Here's how the part is built. I have some questions about the finished solid (model axes, mm). A direction names the side the tool comes from. Coordinates: 2 decimals unless noted, no trailing zeros. Write each loop counter-clockwise with the first axis right and the second up, starting at its lowest first coordinate (ties: lowest second). Pieces come first, ordered by that corner, then holes.
Item 1: For faces 1 (the face through (0.37, 66.05, 0.01)), 2 (the face through (-6.3, 4.7, 12.5)), 3 (the face through (40, 41.5, 0)), which set-ups out of +Z, -Z, +X, -X, +Y, -Y let a thin tool reach every point of the face, with its end or its side?
Item 2: If we section it at B-B (x = -24): Please give me the cut outline in (y, z), then the cut area to 3 significant figures.
Item 3: If I drill on line 1 (Y direction, x = 2.5, z = -5); line 2 (X direction, y = 7, z = -7); line 3 (Y direction, x = -12, z = -1.75), over which ranges is the centre line in solid material (lowest first)?
Item 4: If we section it at D-D (y = 12.5): Please give me the cut outline in (x, z).
Item 5: I'm going to push flat-ended pins straight in: pin 1 Ø8 at (x, z) = (0, 2.5) entering from +Y; pin 2 Ø5 at (y, z) = (59, 0) entering from -X; pin 3 Ø10 at (x, y) = (13, 58.5) entering from +Z. Where does each tip first touch, or does it pass through?
Item 6: We'd pull the mould along Y, two halves only. Please class faces 4 (the face through (41.25, 4, 0)), 5 (the face through (1, 5, 0)), 6 (the face through (-1, 0, 0)): +Y half, -Y half, draft (parallel to the pull), parting line (faces both ways), or undercut.
Item 7: If we section it at C-C (z = -8): Please give me the cut outline in (x, y).
Item 8: If we section it at A-A (x = 0): Please give me the cut outline in (y, z), then the cut area to 3 significant figures.
from build123d import *

# Parameters (mm, degrees)
SKETCH1_W               = 82.5
SKETCH1_H               = 25
BOSS_EXTRUDE1_DEPTH     = 5
SKETCH2_W               = 5
SKETCH2_H               = 25
BOSS_EXTRUDE2_DEPTH     = 39
SKETCH3_W               = 82.5
SKETCH3_H               = 25
BOSS_EXTRUDE3_DEPTH     = 5
BOSS_EXTRUDE4_DEPTH     = 2.5
SKETCH5_W               = 2.5
SKETCH5_H               = 39
BOSS_EXTRUDE5_DEPTH     = 25
CUT_EXTRUDE1_DEPTH      = 86.323912034
CUT_EXTRUDE1_DEPTH_BACK = 25
SKETCH6_W               = 5
SKETCH6_H               = 34
FILLET1_R               = 2
FILLET2_R               = 2


with BuildPart() as part:
    # Sketch1 → Boss-Extrude1 (new body)
    with BuildSketch(Plane(origin=(0, 0, 0), x_dir=(1, 0, 0), z_dir=(0, 1, 0))):
        Rectangle(SKETCH1_W, SKETCH1_H)
    extrude(amount=BOSS_EXTRUDE1_DEPTH)

    # Sketch2 → Boss-Extrude2 (add)
    with BuildSketch(Plane(origin=(0, 5, 0), x_dir=(1, 0, 0), z_dir=(0, 1, 0))):
        with Locations((-38.75, 0)):
            Rectangle(SKETCH2_W, SKETCH2_H)
    extrude(amount=BOSS_EXTRUDE2_DEPTH)

    # Sketch3 → Boss-Extrude3 (add)
    with BuildSketch(Plane(origin=(0, 44, 0), x_dir=(1, 0, 0), z_dir=(0, 1, 0))):
        Rectangle(SKETCH3_W, SKETCH3_H)
    extrude(amount=BOSS_EXTRUDE3_DEPTH)

    # Sketch4 → Boss-Extrude4 (add, symmetric)
    with BuildSketch(Plane.XY):
        with BuildLine():
            Line((-17.053024247, 49), (-21.381868864, 49))
            ThreePointArc((-21.381868864, 49), (0, 70.381868864), (21.381868864, 49))
            Line((21.381868864, 49), (17.053024247, 49))
            ThreePointArc((17.053024247, 49), (0, 66.053024247), (-17.053024247, 49))
        make_face()
    extrude(amount=BOSS_EXTRUDE4_DEPTH, both=True)

    # Sketch5 → Boss-Extrude5 (add)
    with BuildSketch(Plane.XY.offset(12.5)):
        with Locations((40, 24.5)):
            Rectangle(SKETCH5_W, SKETCH5_H)
    extrude(amount=-BOSS_EXTRUDE5_DEPTH)

    # Sketch6 → Cut-Extrude1 (cut, two sides: drawn at the far end of the back side and taken through both)
    with BuildSketch(Plane.XY.offset(12.5).offset(-CUT_EXTRUDE1_DEPTH_BACK)):
        with Locations((38.75, 24.5)):
            Rectangle(SKETCH6_W, SKETCH6_H)
    extrude(amount=CUT_EXTRUDE1_DEPTH + CUT_EXTRUDE1_DEPTH_BACK, mode=Mode.SUBTRACT)

    # Fillet1
    fillet1_edges = [part.edges().sort_by_distance(p)[0] for p in [
        (0, 70.381868864, -2.5),
        (0, 70.381868864, 2.5),
    ]]
    fillet(fillet1_edges, radius=FILLET1_R)

    # Fillet2
    fillet2_edges = [part.edges().sort_by_distance(p)[0] for p in [
        (0, 66.053024247, -2.5),
        (0, 66.053024247, 2.5),
    ]]
    fillet(fillet2_edges, radius=FILLET2_R)


solid = part.part
Answer list:
1. face 1: +Z, -Z
1. face 2: +Z, +X, -X, +Y, -Y
1. face 3: +Z, -Z, +X
2. outline: (0, -12.5) - (5, -12.5) - (5, 12.5) - (0, 12.5) - close; (44, -12.5) - (49, -12.5) - (49, 12.5) - (44, 12.5) - close
2. area: 250 mm2
3. line 1: y = 0 to 5, 44 to 49
3. line 2: x = -41.25 to -36.25, 38.75 to 41.25
3. line 3: y = 0 to 5, 44 to 49, 61.73 to 66.16
4. outline: (-41.25, -12.5) - (-36.25, -12.5) - (-36.25, 12.5) - (-41.25, 12.5) - close
5. pin 1: stops at y = 70.38
5. pin 2: stops at x = -20.02
5. pin 3: stops at z = 2.5
6. face 4: draft
6. face 5: undercut
6. face 6: -Y half
7. outline: (-41.25, 0) - (41.25, 0) - (41.25, 7.5) - (38.75, 7.5) - (38.75, 5) - (-36.25, 5) - (-36.25, 44) - (38.75, 44) - (38.75, 41.5) - (41.25, 41.5) - (41.25, 49) - (-41.25, 49) - close
8. outline: (0, -12.5) - (5, -12.5) - (5, 12.5) - (0, 12.5) - close; (44, -12.5) - (49, -12.5) - (49, 12.5) - (44, 12.5) - close; (66.05, -0.5) arc R2 ccw to (68.05, -2.5) - (68.38, -2.5) arc R2 ccw to (70.38, -0.5) - (70.38, 0.5) arc R2 ccw to (68.38, 2.5) - (68.05, 2.5) arc R2 ccw to (66.05, 0.5) - close
8. area: 268 mm2
